Build history of the part. All positions in model axes, mm. Face numbers are marked on the shaded views. A direction names the side the tool comes from. Give positions to 0.01 mm unless a question says otherwise; leave off trailing zeros. Loops run counter-clockwise (first coordinate to the right, second up) from the corner with the lowest first, then second, coordinate; pieces in that order, holes last. Notation, with made-up numbers: (31, 26) - (65, 26) arc R13 cw to (65, 35) - close; hole circle Ø7 at (82.25, 27.25). An arc over 180 degrees is marked (long way). Return JSON: item names as keys, results as strings. Group by question number.
1) 3-axis set-ups, long thin cutter, end or side, ignore diameter. For the marked faces 4, 5, 6, 7 and 8: which of +Z, -Z, +X, -X, +Y, -Y reach the whole face in a straight line?
2) Drop flat-ended pins along their axis: pin 1 (10 mm diameter, centred on x = -4.5, z = -2.5, fed in from +Y) (3 decimals); pin 2 (1.5 mm diameter, centred on y = 3, z = 1, fed in from -X); pin 3 (1.6 mm diameter, centred on y = 1.5, z = 0, fed in from +X). Give the stop position or say it passes through.
3) Slice it at A-A (x = -11.75). List the corners of the cut face in (y, z) (3 decimals), and give its area (3 significant figures).
4) Mould opens along Z. For the marked faces 1, 2 and 3 say: released by +Z, released by -Z, zero draft, split by the parting line, or undercut.
5) Drill centre lines: probe 1 along X at (y, z) = (1.5, 6.5); probe 2 along X at (y, z) = (1.9, 3); probe 3 along Z at (x, y) = (13, 2.1) (3 decimals). Where is each one in solid material? Low to high. Write a range as from..to.
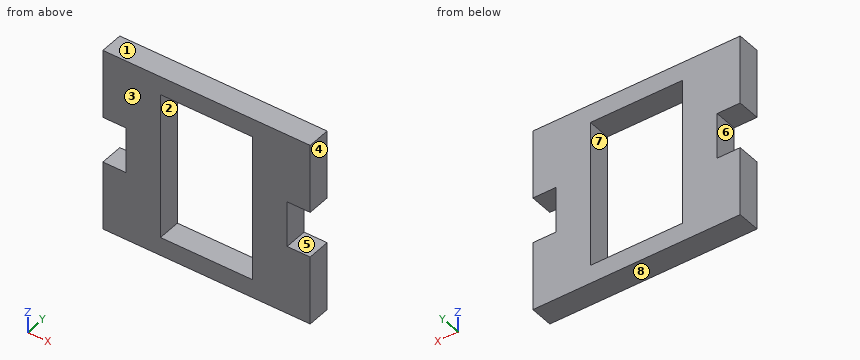
```python
from build123d import *

# Parameters (mm, degrees)
SKETCH1_W           = 12.7
SKETCH1_H           = 20.32
BOSS_EXTRUDE1_DEPTH = 3.175


with BuildPart() as part:
    # Sketch1 → Boss-Extrude1 (new body)
    with BuildSketch(Plane(origin=(0, 0, 0), x_dir=(1, 0, 0), z_dir=(0, 1, 0))):
        Polygon((-14.2875, 3.175), (-11.1125, 3.175), (-11.1125, -3.175), (-14.2875, -3.175), (-14.2875, -12.7), (14.2875, -12.7), (14.2875, -3.175), (11.1125, -3.175), (11.1125, 3.175), (14.2875, 3.175), (14.2875, 12.7), (-14.2875, 12.7), align=None)
        Rectangle(SKETCH1_W, SKETCH1_H, mode=Mode.SUBTRACT)
    extrude(amount=BOSS_EXTRUDE1_DEPTH)


solid = part.part
```
Results:
{
 "1": {"face 4": "+Z, -Z, +X, +Y, -Y", "face 5": "+X, +Y, -Y", "face 6": "-X, +Y, -Y", "face 7": "+Y, -Y", "face 8": "-Z, +X, -X, +Y, -Y"},
 "2": {"pin 1": "y = 3.175", "pin 2": "x = -11.11", "pin 3": "x = 11.11"},
 "3": {"outline": "(0, -12.7) - (3.175, -12.7) - (3.175, -3.175) - (0, -3.175) - close; (0, 3.175) - (3.175, 3.175) - (3.175, 12.7) - (0, 12.7) - close", "area": "60.5 mm2"},
 "4": {"face 1": "released by +Z", "face 2": "undercut", "face 3": "zero draft"},
 "5": {"probe 1": "-14.29..-6.35, 6.35..14.29", "probe 2": "-11.11..-6.35, 6.35..11.11", "probe 3": "-12.7..-3.175, 3.175..12.7"}
}
